Here's the drawing with two shaded views (mm, measured from the low corner). I have some questions. Round coordinates to 2 decimals unless told otherwise and drop trailing zeros. Order: outer loops, then holes, each group sorted by start corner. A loop starts at its lowest first (then second) coordinate and runs counter-clockwise, first axis right, second up. Notation, with made-up numbers: M -16,-33 L 20,-33 A3 cw 20,-29 Z; hole C 78.25,-1.75 d2. An arc over 180 degrees is marked long. One line per question, with ' | ' between items.
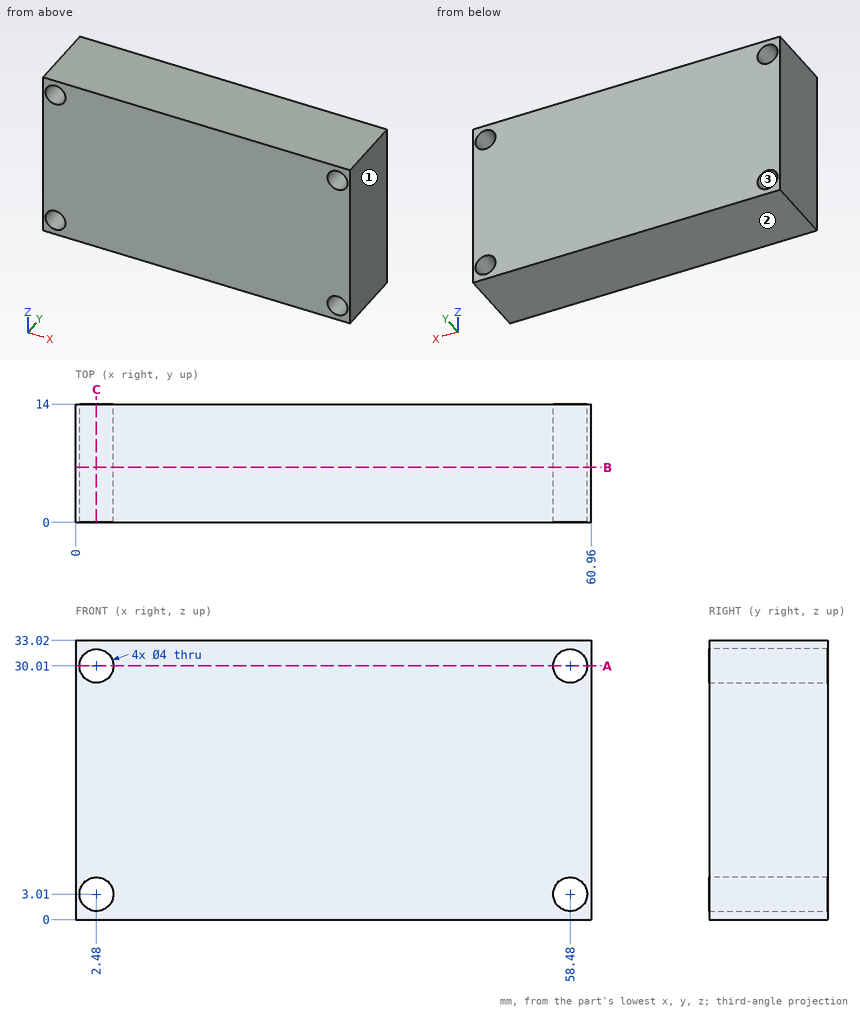
(1) Will this pin go through, and if not, where does the flat tip stop? pin 1 Ø3 at (x, z) = (58.48, 30.01) entering from -Y.
Final values:
pin 1: through
(2) If we section it at C-C on x = 2.48: Please give me the cut outline in (y, z), plus the area to 3 significant figures.
Final values:
outline: M 0,0 L 14,0 L 14,1.01 L 0,1.01 Z; M 0,5.01 L 14,5.01 L 14,28.01 L 0,28.01 Z; M 0,32.01 L 14,32.01 L 14,33.02 L 0,33.02 Z | area: 350 mm^2
(3) Please list where these lines run through material, in increasing order: probe 1 along X at (y, z) = (7, 30.01); probe 2 along X at (y, z) = (7.5, 4). Write a range as [from, to].
Final values:
probe 1: [0, 0.48], [4.48, 56.48], [60.48, 60.96] | probe 2: [0, 0.74], [4.22, 56.74], [60.22, 60.96]
(4) If we section it at B-B on y = 6.5: Please give me the cut outline in (x, z).
Final values:
outline: M 0,0 L 60.96,0 L 60.96,33.02 L 0,33.02 Z; hole C 2.48,3.01 d4; hole C 2.48,30.01 d4; hole C 58.48,3.01 d4; hole C 58.48,30.01 d4
(5) If we section it at A-A on z = 30.01: Please give me the cut outline in (x, y).
Final values:
outline: M 0,0 L 0.48,0 L 0.48,14 L 0,14 Z; M 4.48,0 L 56.48,0 L 56.48,14 L 4.48,14 Z; M 60.48,0 L 60.96,0 L 60.96,14 L 60.48,14 Z
(6) Thinking about a two-plate mould opening in X: for the marked faces 1, 2 and 3, which applies, released by +X, released by -X, zero draft, split by the parting line, or undercut?
Final values:
face 1: released by +X | face 2: zero draft | face 3: undercut
